The listing builds one solid part. Answer for the finished solid, in the listing's coordinates (mm). Face numbers are marked on the shaded views. Round coordinates to 2 decimals unless told otherwise and drop trailing zeros. Write each loop counter-clockwise with the first axis right and the second up, starting at its lowest first coordinate (ties: lowest second). Pieces come first, ordered by that corner, then holes. Notation, with made-up numbers: M 76,23 L 124,23 A19 cw 124,34 Z; hole C 87.25,-38 d9. An arc over 180 degrees is marked long. Write each question's results on one line, items separated by ' | '.
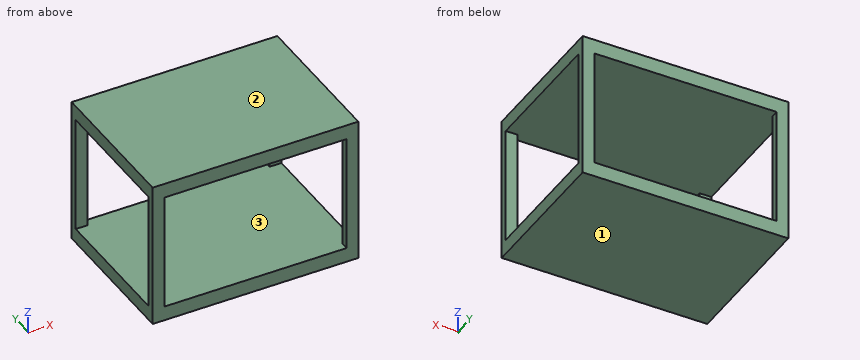
from build123d import *

# Parameters (mm, degrees)
F0_W     = 700
F0_H     = 500
F1_DEPTH = 500
F2_W     = 620
F2_H     = 400
F3_DEPTH = 810
F4_W     = 450
F4_H     = 400
F5_DEPTH = 777


with BuildPart() as f1:
    # F0 (on Top) → F1 (new body)
    with BuildSketch(Plane.XY):
        Rectangle(F0_W, F0_H)
    extrude(amount=F1_DEPTH)

    # F2 (on face) → F3 (cut)
    with BuildSketch(Plane.XZ.offset(250)):
        with Locations((0, 250)):
            Rectangle(F2_W, F2_H)
    extrude(amount=-F3_DEPTH, mode=Mode.SUBTRACT)

    # F4 (on face) → F5 (cut)
    with BuildSketch(Plane(origin=(-350, 0, 0), x_dir=(0, -1, 0), z_dir=(-1, 0, 0))):
        with Locations((0, 250)):
            Rectangle(F4_W, F4_H)
    extrude(amount=-F5_DEPTH, mode=Mode.SUBTRACT)


solid = f1.part
1) Section A-A (x = -24) is taken. Determine the outline of the cut face in (y, z).
Return value:
outline: M -250,0 L 250,0 L 250,50 L -250,50 Z; M -250,450 L 250,450 L 250,500 L -250,500 Z
2) Section B-B (y = -159) is taken. Determine the outline of the cut face in (x, z), then the cut area to 3 significant figures.
Return value:
outline: M -350,0 L 350,0 L 350,50 L -350,50 Z; M -350,450 L 350,450 L 350,500 L -350,500 Z | area: 70,000 mm²
3) Section C-C (z = 240.5) is taken. Determine the outline of the cut face in (x, y), then the cut area to 3 significant figures.
Return value:
outline: M -350,-250 L -310,-250 L -310,-225 L -350,-225 Z; M -350,225 L -310,225 L -310,250 L -350,250 Z; M 310,-250 L 350,-250 L 350,-225 L 310,-225 Z; M 310,225 L 350,225 L 350,250 L 310,250 Z | area: 4,000 mm²
4) Find the intervals of material crossed by line 1 (Z direction, x = -105, y = 34.5), in increasing order.
Return value:
line 1: 0 to 50, 450 to 500
5) The mould has two halves that part along Z. Classify the marked faces 1, 2 and 3: +Z half, -Z half, draft (parallel to the pull), parting line (faces both ways), or undercut.
Return value:
face 1: -Z half | face 2: +Z half | face 3: undercut
